```python
from build123d import *

# Parameters (mm, degrees)
SKETCH1_R           = 31.5
BOSS_EXTRUDE1_DEPTH = 25
SKETCH3_R           = 2.5
CUT_EXTRUDE1_DEPTH  = 25
SHELL1_T            = -10


with BuildPart() as part:
    # Sketch1 → Boss-Extrude1 (new body)
    with BuildSketch(Plane(origin=(0, 0, 0), x_dir=(0, 0, -1), z_dir=(1, 0, 0))):
        Circle(SKETCH1_R)
    extrude(amount=BOSS_EXTRUDE1_DEPTH)

    # Sketch3 → Cut-Extrude1 (cut)
    with BuildSketch(Plane.ZY):
        Circle(SKETCH3_R)
    extrude(amount=-CUT_EXTRUDE1_DEPTH, mode=Mode.SUBTRACT)

    # Shell1
    shell1_openings = [part.faces().sort_by_distance(p)[0] for p in [
        (25, 0, 2.5),
    ]]
    offset(amount=SHELL1_T, openings=shell1_openings, kind=Kind.INTERSECTION)


solid = part.part
```
Source: CAD feature listing. Evaluate the final solid. Frame: model axes, mm. A direction names the side the tool comes from. Give positions to 0.01 mm unless a question says otherwise; leave off trailing zeros. Order: outer loops, then holes, each group sorted by start corner. A loop starts at its lowest first (then second) coordinate and runs counter-clockwise, first axis right, second up.
(1) Contact query for flat-ended pins moving along their axis: P1, Ø1, axis at x = 5.5, z = 0.5, coming from the -Y side; P2, Ø2, axis at x = 8, y = 1.5, coming from the -Z side; P3, Ø5, axis at x = 16.5, y = -4.5, coming from the -Z side. Output: stop coordinate, or through.
(2) Section query D-D (y = -14.5). Return the cut outline in (x, z).
(3) Access query for faces 4 (the face through (10, -9, -9)), 5 (the face through (25, -7, -21)). Directions: +Z, -Z, +X, -X, +Y, -Y. A direction counts if a zero-diameter tool reaches every point of the face in a straight line with its end or side. Return the directions, or none.
(4) Pull-direction query (Z, two-part tool) for faces 1 (the face through (25, -3, 0)), 2 (the face through (17.395, 3.755, 11.923)), 3 (the face through (12.325, 31.232, 4.101)); classes: +Z half, -Z half, draft (parallel to the pull), parting line (faces both ways), or undercut.
(5) Section query A-A (y = 0). Return the cut outline in (x, z).
(6) Material intervals for line 1 along Y through (x, z) = (14.5, 0); line 2 along Y through (x, z) = (24.25, -3); line 3 along Y through (x, z) = (15.75, -7.5), sorted ascending.
(7) Section query C-C (x = 20.5). Return the cut outline in (y, z), plus the area to 3 significant figures.
Outcome:
1. P1: stops at y = -31.5
1. P2: stops at z = -31.5
1. P3: stops at z = -31.44
2. outline: (0, -27.96) - (25, -27.96) - (25, -15.87) - (10, -15.87) - (10, 15.87) - (25, 15.87) - (25, 27.96) - (0, 27.96) - close
3. face 4: +X
3. face 5: +Z, -Z, +X, +Y, -Y
4. face 1: draft
4. face 2: undercut
4. face 3: parting line
5. outline: (0, -31.5) - (25, -31.5) - (25, -21.5) - (10, -21.5) - (10, -12.5) - (25, -12.5) - (25, -2.5) - (0, -2.5) - close; (0, 2.5) - (25, 2.5) - (25, 12.5) - (10, 12.5) - (10, 21.5) - (25, 21.5) - (25, 31.5) - (0, 31.5) - close
6. line 1: y = -31.5 to -21.5, -12.5 to -2.5, 2.5 to 12.5, 21.5 to 31.5
6. line 2: y = -31.36 to -21.29, -12.13 to 12.13, 21.29 to 31.36
6. line 3: y = -30.59 to -20.15, -10 to 10, 20.15 to 30.59
7. outline: circle Ø63 at (0, 0); circle Ø25 at (0, 0); hole circle Ø43 at (0, 0); hole circle Ø5 at (0, 0)
7. area: 2,140 mm2
